```python
from build123d import *

# Parameters (mm, degrees)
SKETCH1_W           = 50.8
SKETCH1_H           = 63.5
BOSS_EXTRUDE1_DEPTH = 7.62
FILLET1_R           = 12.7


with BuildPart() as part:
    # Sketch1 → Boss-Extrude1 (new body)
    with BuildSketch(Plane.XY):
        with BuildLine():
            Line((0, 0), (-88.9, 0))
            ThreePointArc((-88.9, 0), (-114.3, 19.05), (-139.7, 0))
            Line((-139.7, 0), (-228.6, 0))
            Line((-228.6, 0), (-228.6, 101.6))
            Line((-228.6, 101.6), (-139.7, 101.6))
            ThreePointArc((-139.7, 101.6), (-114.3, 82.55), (-88.9, 101.6))
            Line((-88.9, 101.6), (0, 101.6))
            Line((0, 101.6), (0, 0))
        make_face()
        with Locations((-184.15, 50.8)):
            Rectangle(SKETCH1_W, SKETCH1_H, mode=Mode.SUBTRACT)
        with Locations((-44.45, 50.8)):
            Rectangle(SKETCH1_W, SKETCH1_H, mode=Mode.SUBTRACT)
    extrude(amount=BOSS_EXTRUDE1_DEPTH)

    # Fillet1
    fillet1_edges = [part.edges().sort_by_distance(p)[0] for p in [
        (0, 0, 3.81),
        (-88.9, 0, 3.81),
        (-139.7, 0, 3.81),
        (-228.6, 0, 3.81),
        (-228.6, 101.6, 3.81),
        (-139.7, 101.6, 3.81),
        (-88.9, 101.6, 3.81),
        (0, 101.6, 3.81),
    ]]
    fillet(fillet1_edges, radius=FILLET1_R)


solid = part.part
```
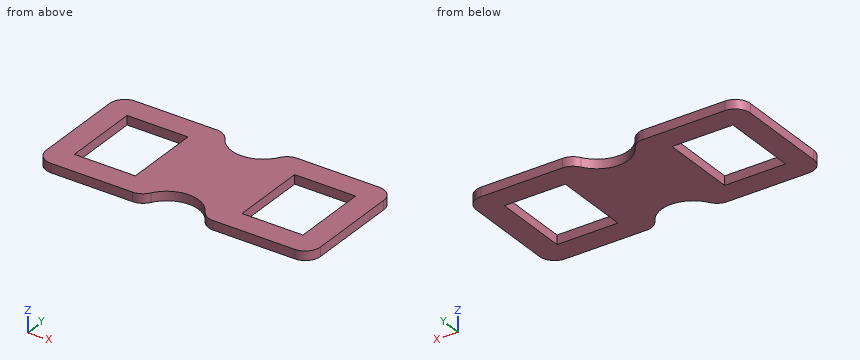
Source: CAD feature listing. Evaluate the final solid. Frame: model axes, mm. Coordinates: 2 decimals unless noted, no trailing zeros. Loops run counter-clockwise (first coordinate to the right, second up) from the corner with the lowest first, then second, coordinate; pieces in that order, holes last. Notation, with made-up numbers: M 4,-21.5 L 37,-21.5 A37 ccw 37,17.5 Z; hole C 84.25,-29 d8. An arc over 180 degrees is marked long. Put each result on its own line as item: value. Start each with the question number.
1) Ray query, L1, parallel to X at y = 54.5, z = 2.5; L2, parallel to Y at x = -20, z = 5.25; L3, parallel to X at y = 96.5, z = 4.5. Return the intervals inside material, ascending. Write a range as from..to.
2) Contact query for a flat-ended pin moving along its axis: pin 1 Ø3 at (x, y) = (-48, 20.5) entering from +Z. Output: stop coordinate, or through.
3) Cut plane C-C on y = 38. Return the cut outline in (x, z).
4) Cut plane A-A on z = 2.5. Return the cut outline in (x, y), then the cut area to 3 significant figures.
5) Cut plane B-B on x = -40. Return the cut outline in (y, z), then the cut area to 3 significant figures.
The answers:
1. L1: x = -228.6..-209.55, -158.75..-69.85, -19.05..0
1. L2: y = 0..19.05, 82.55..101.6
1. L3: x = -226.07..-137.73, -90.87..-2.53
2. pin 1: stops at z = 7.62
3. outline: M -228.6,0 L -209.55,0 L -209.55,7.62 L -228.6,7.62 Z; M -158.75,0 L -69.85,0 L -69.85,7.62 L -158.75,7.62 Z; M -19.05,0 L 0,0 L 0,7.62 L -19.05,7.62 Z
4. outline: M -228.6,12.7 A12.7 ccw -215.9,0 L -147.9,0 A12.7 ccw -137,6.18 A26.46 cw -91.6,6.18 A12.7 ccw -80.7,0 L -12.7,0 A12.7 ccw 0,12.7 L 0,88.9 A12.7 ccw -12.7,101.6 L -80.7,101.6 A12.7 ccw -91.6,95.42 A26.46 cw -137,95.42 A12.7 ccw -147.9,101.6 L -215.9,101.6 A12.7 ccw -228.6,88.9 Z; hole M -209.55,19.05 L -158.75,19.05 L -158.75,82.55 L -209.55,82.55 Z; hole M -69.85,19.05 L -19.05,19.05 L -19.05,82.55 L -69.85,82.55 Z
4. area: 15,200 mm²
5. outline: M 0,0 L 19.05,0 L 19.05,7.62 L 0,7.62 Z; M 82.55,0 L 101.6,0 L 101.6,7.62 L 82.55,7.62 Z
5. area: 290 mm²
